Here's how the part is built. I have some questions about the finished solid (model axes, mm). Face numbers are marked on the shaded views. A direction names the side the tool comes from. Round coordinates to 2 decimals unless told otherwise and drop trailing zeros. Write each loop counter-clockwise with the first axis right and the second up, starting at its lowest first coordinate (ties: lowest second). Pieces come first, ordered by that corner, then holes. Notation, with made-up numbers: (-13, 35.5) - (26, 35.5) arc R17 ccw to (26, 53.5) - close; hole circle Ø5 at (54, 30.5). An arc over 180 degrees is marked (long way). One line per item, written item: value. Start each with the question number.
Item 1: Imagine slicing it at C-C, the plane x = -43.5. Please give me the cut outline in (y, z), then the cut area to 3 significant figures.
Item 2: For P1, Ø6, axis at x = 40.5, z = 17, coming from the -Y side; P2, Ø4, axis at x = -31.5, z = 2, coming from the +Y side, each with a flat end and sliding along its axis, tell me the tip position at first contact or that it passes through.
Item 3: Thinking about a two-plate mould opening in Y: for the marked faces 4, 5 and 6, which applies, released by +Y, released by -Y, zero draft, split by the parting line, or undercut?
Item 4: Imagine slicing it at B-B, the plane y = 0. Please give me the cut outline in (x, z).
Item 5: Imagine slicing it at D-D, the plane z = 9. Please give me the cut outline in (x, y).
Item 6: If I drill on line 1 (X direction, y = -8.5, z = -15); line 2 (X direction, y = -5.5, z = -18); line 3 (Y direction, x = 1.5, z = -19), over which ranges is the centre line in solid material (lowest first)?
Item 7: Imagine slicing it at A-A, the plane z = 23.5. Please give me the cut outline in (x, y), then the cut area to 3 significant figures.
Item 8: For the marked faces 1, 2 and 3, which set-ups out of +Z, -Z, +X, -X, +Y, -Y let a thin tool reach every point of the face, with its end or its side?
```python
from build123d import *

# Parameters (mm, degrees)
F1_DEPTH = 50
F2_DEPTH = 50
F3_DEPTH = 65
F4_DEPTH = 65
F5_R     = 10
F6_DEPTH = 200


with BuildPart() as f1:
    # F0 (on Front) → F1 (new body)
    with BuildSketch(Plane.XZ):
        with BuildLine():
            Line((60, 35), (35, 35))
            ThreePointArc((35, 35), (24.7487373415, 10.2512626585), (0, 0))
            Line((0, 0), (0, -35))
            Line((0, -35), (60, -35))
            Line((60, -35), (60, 35))
        make_face()
    extrude(amount=F1_DEPTH)

    # F2 (add): a face of the model
    f2_faces = [f1.faces().sort_by_distance(p)[0] for p in [
        (34.5003777815, 0, -5.9860884872),
    ]]
    extrude(f2_faces, amount=F2_DEPTH)

    # F0 (on Front) → F3 (join)
    with BuildSketch(Plane.XZ):
        with BuildLine():
            Line((35, 35), (17.5, 35))
            ThreePointArc((17.5, 35), (12.3743686708, 22.6256313292), (0, 17.5))
            Line((0, 17.5), (0, 0))
            ThreePointArc((0, 0), (24.7487373415, 10.2512626585), (35, 35))
        make_face()
    extrude(amount=F3_DEPTH)

    # F4 (add): a face of the model
    f4_faces = [f1.faces().sort_by_distance(p)[0] for p in [
        (17.3302049145, 0, 17.6697950855),
    ]]
    extrude(f4_faces, amount=F4_DEPTH)

    # F5 (on face) → F6 (cut)
    with BuildSketch(Plane.XY.offset(35)):
        with Locations((47.3726391792, 0)):
            Circle(F5_R)
    extrude(amount=-F6_DEPTH, mode=Mode.SUBTRACT)

    # F7: F1 across face


with BuildPart() as f1_1:
    add(f1.part)
    add(f1.part.mirror(Plane(origin=(0, 0, -7.1590909091), x_dir=(0, -1, 0), z_dir=(-1, 0, 0))))


solid = f1_1.part
```
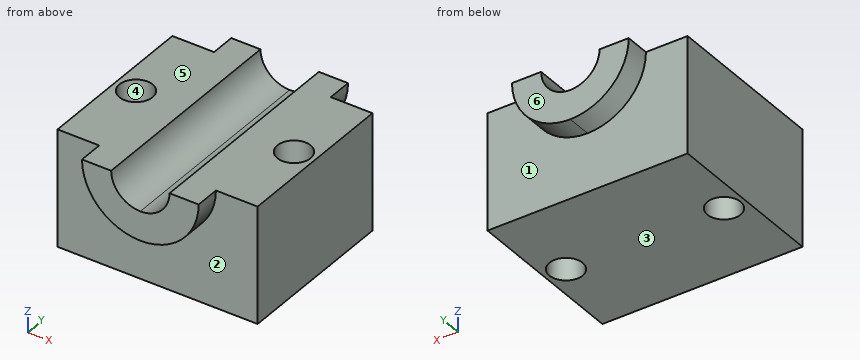
Values follow:
1. outline: (-50, -35) - (-9.22, -35) - (-9.22, 35) - (-50, 35) - close; (9.22, -35) - (50, -35) - (50, 35) - (9.22, 35) - close
1. area: 5,710 mm^2
2. P1: stops at y = -50
2. P2: stops at y = 50
3. face 4: undercut
3. face 5: zero draft
3. face 6: released by +Y
4. outline: (-60, -35) - (-57.37, -35) - (-57.37, 35) - (-60, 35) - close; (-37.37, -35) - (37.37, -35) - (37.37, 35) - (17.5, 35) arc R17.5 cw to (-17.5, 35) - (-37.37, 35) - close; (57.37, -35) - (60, -35) - (60, 35) - (57.37, 35) - close
5. outline: (-60, -50) - (-23.43, -50) - (-23.43, -65) - (23.43, -65) - (23.43, -50) - (60, -50) - (60, 50) - (23.43, 50) - (23.43, 65) - (-23.43, 65) - (-23.43, 50) - (-60, 50) - close; hole circle Ø20 at (-47.37, 0); hole circle Ø20 at (47.37, 0)
6. line 1: x = -60 to -52.64, -42.1 to 42.1, 52.64 to 60
6. line 2: x = -60 to -55.72, -39.02 to 39.02, 55.72 to 60
6. line 3: y = -50 to 50
7. outline: (-60, -50) - (-33.06, -50) - (-33.06, -65) - (-13.19, -65) - (-13.19, 65) - (-33.06, 65) - (-33.06, 50) - (-60, 50) - close; (13.19, -65) - (33.06, -65) - (33.06, -50) - (60, -50) - (60, 50) - (33.06, 50) - (33.06, 65) - (13.19, 65) - close; hole circle Ø20 at (-47.37, 0); hole circle Ø20 at (47.37, 0)
7. area: 9,930 mm^2
8. face 1: -Z, +Y
8. face 2: -Z, -Y
8. face 3: -Z, +X, -X, +Y, -Y
